Could you check a few things on this model? Use its own coordinates, in mm. Face numbers are marked on the shaded views. A direction names the side the tool comes from. Coordinates: 2 decimals unless noted, no trailing zeros. Write each loop counter-clockwise with the first axis right and the second up, starting at its lowest first coordinate (ties: lowest second). Pieces come first, ordered by that corner, then holes.
```python
from build123d import *

# Parameters (mm, degrees)
BOSS_EXTRUDE1_DEPTH       = 100
FILLET1_R                 = 20
FILLET2_R                 = 20
CUT_EXTRUDE1_DEPTH        = 13
F_1_0MM_DOWEL_HOLE1_D     = 8
F_1_0MM_DOWEL_HOLE1_DEPTH = 12.596557524
F_1_0MM_DOWEL_HOLE1_TIP   = 2.403442476


with BuildPart() as part:
    # Sketch3 → Boss-Extrude1 (new body)
    with BuildSketch(Plane(origin=(0, 0, 0), x_dir=(0, 0, -1), z_dir=(1, 0, 0))):
        Polygon((24.06709422, 65), (0, 0), (13.862503416, 0), (37.929597637, 65), align=None)
        with BuildLine():
            Line((25.203655824, 68.069606309), (24.06709422, 65))
            Line((24.06709422, 65), (37.929597637, 65))
            Line((37.929597637, 65), (39.796344176, 70.041677401))
            ThreePointArc((39.796344176, 70.041677401), (40.895779886, 71.46221772), (42.609688839, 72))
            Line((42.609688839, 72), (45, 72))
            Line((45, 72), (45, 80))
            Line((45, 80), (20, 80))
            Line((20, 80), (20, 72.11128371))
            Line((20, 72.11128371), (22.390311161, 72.11128371))
            ThreePointArc((22.390311161, 72.11128371), (24.852528882, 70.825192663), (25.203655824, 68.069606309))
        make_face()
    extrude(amount=BOSS_EXTRUDE1_DEPTH)

    # Fillet1
    fillet1_edges = [part.edges().sort_by_distance(p)[0] for p in [
        (100, 0, -6.931251708),
    ]]
    fillet(fillet1_edges, radius=FILLET1_R)

    # Fillet2
    fillet2_edges = [part.edges().sort_by_distance(p)[0] for p in [
        (0, 0, -6.931251708),
    ]]
    fillet(fillet2_edges, radius=FILLET2_R)

    # Sketch4 → Cut-Extrude1 (cut)
    with BuildSketch(Plane(origin=(0, 0, 0), x_dir=(1, 0, 0), z_dir=(0, 0.34722580038254636, 0.9377815542804733))):
        with BuildLine():
            Line((10, 66.96704035), (10, 20))
            ThreePointArc((10, 20), (12.928932188, 12.928932188), (20, 10))
            Line((20, 10), (80, 10))
            ThreePointArc((80, 10), (87.071067812, 12.928932188), (90, 20))
            Line((90, 20), (90, 66.96704035))
            Line((90, 66.96704035), (10, 66.96704035))
        make_face()
    extrude(amount=-CUT_EXTRUDE1_DEPTH, mode=Mode.SUBTRACT)

    # Ø1.0mm Dowel Hole1
    with Locations(Plane(origin=(0, 80, 0), x_dir=(1, 0, 0), z_dir=(0, 1, 0))):
        with Locations((25, 32.5), (75, 32.5)):
            Hole(F_1_0MM_DOWEL_HOLE1_D / 2, depth=F_1_0MM_DOWEL_HOLE1_DEPTH)
            with Locations((0, 0, -(F_1_0MM_DOWEL_HOLE1_DEPTH + F_1_0MM_DOWEL_HOLE1_TIP / 2))):  # 118° drill point
                Cone(0, F_1_0MM_DOWEL_HOLE1_D / 2, F_1_0MM_DOWEL_HOLE1_TIP, mode=Mode.SUBTRACT)


solid = part.part
```
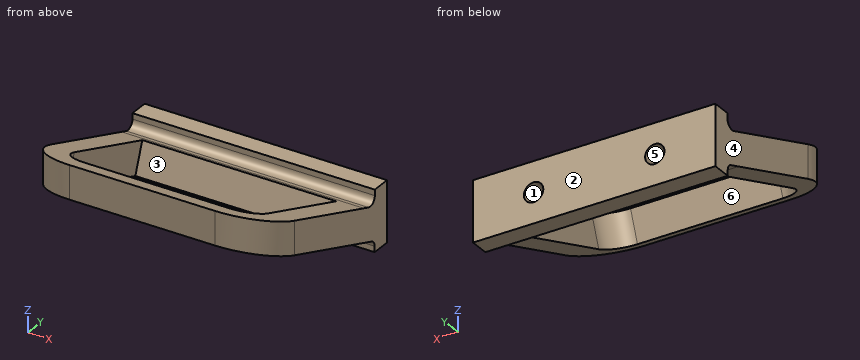
Item 1: I want a section at C-C, the plane x = 85.5. List the corners of the cut face in (y, z) for me, then the cut area to 3 significant figures.
Item 2: If I drill on line 1 along X through (y, z) = (76, -32.5); line 2 along Z through (x, y) = (25, 72.5); line 3 along X through (y, z) = (28, -15), over which ranges is the centre line in solid material (lowest first)?
Item 3: Which directions (+Z, -Z, +X, -X, +Y, -Y) give clear straight access to the entire face, cutting with the end or side of a thin tool? Please do the marked faces 4, 5 and 6.
Item 4: If we mould it in two halves opening along Z, with no side actions, what happens to the marked faces 1, 2 and 3? For each: released by +Z, released by -Z, zero draft, split by the parting line, or undercut.
Item 5: I want a section at B-B, the plane y = 34.5. List the corners of the cut face in (x, z) for me, then the cut area to 3 significant figures.
Item 6: Will these pins go through, and if not, where does the flat tip stop? pin 1 Ø1.2 at (x, z) = (40.5, -43.5) entering from -Y; pin 2 Ø9 at (x, z) = (25, -32.5) entering from -Y; pin 3 Ø6.5 at (x, y) = (27.5, 74.5) entering from +Z; pin 4 Ø4 at (y, z) = (19.5, -11) entering from -X.
Item 7: I want a section at A-A, the plane x = 55.5. List the corners of the cut face in (y, z) for me.
Taken from the geometry:
1. outline: (0.77, -14.15) - (6.41, -16.24) - (10.92, -4.04) - (0.77, -0.29) - close; (58.29, -35.44) - (70.04, -39.8) arc R3 cw to (72, -42.61) - (72, -45) - (80, -45) - (80, -20) - (72.11, -20) - (72.11, -22.39) arc R3 cw to (68.07, -25.2) - (62.8, -23.25) - close
1. area: 473 mm2
2. line 1: x = 0 to 21, 29 to 71, 79 to 100
2. line 2: z = -45 to -36.5, -28.5 to -20
2. line 3: x = 0 to 10, 90 to 100
3. face 4: +Z, -Z, -X, +Y, -Y
3. face 5: +Y
3. face 6: -Z, +Y
4. face 1: undercut
4. face 2: zero draft
4. face 3: released by +Z
5. outline: (0, -26.64) - (10, -26.64) - (10, -12.77) - (0, -12.77) - close; (90, -26.64) - (100, -26.64) - (100, -12.77) - (90, -12.77) - close
5. area: 277 mm2
6. pin 1: stops at y = 72
6. pin 2: stops at y = 58.29
6. pin 3: stops at z = -20
6. pin 4: stops at x = 0
7. outline: (0, -13.86) - (4.86, -15.66) - (9.38, -3.47) - (0, 0) - close; (58.29, -35.44) - (70.04, -39.8) arc R3 cw to (72, -42.61) - (72, -45) - (80, -45) - (80, -20) - (72.11, -20) - (72.11, -22.39) arc R3 cw to (68.07, -25.2) - (62.8, -23.25) - close
